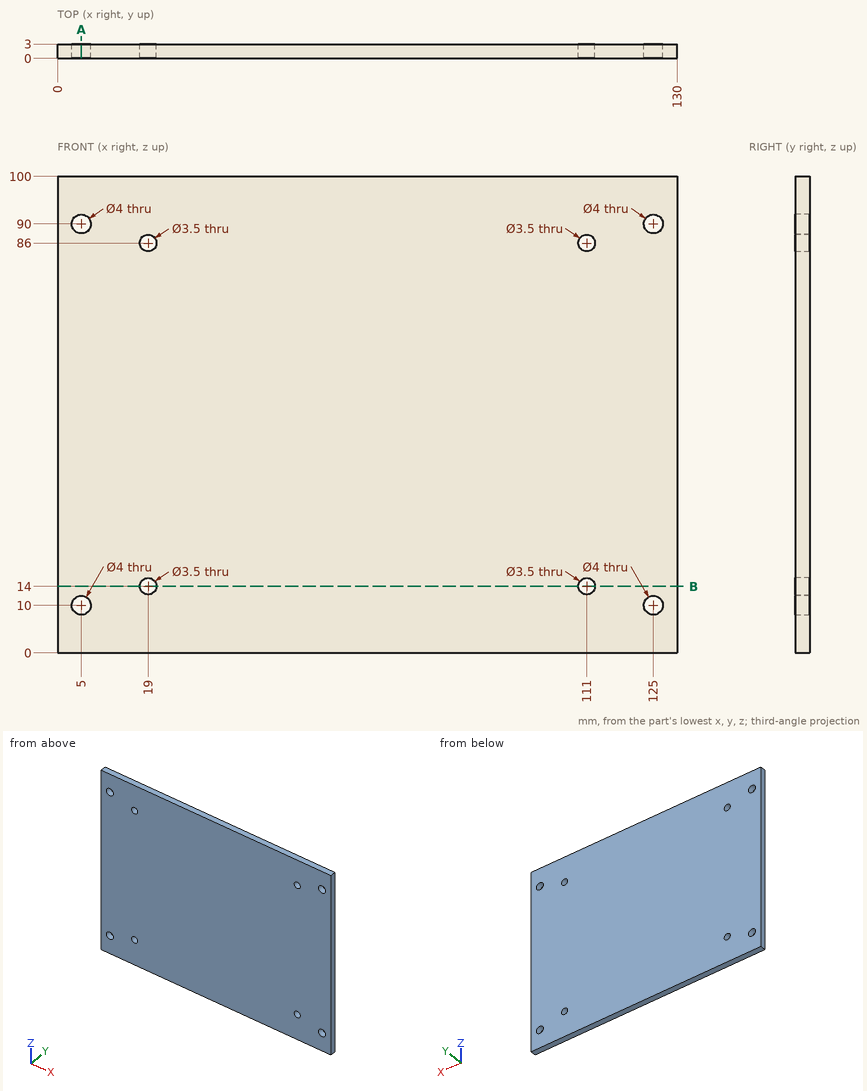
Check sheet for the drawn part. Datum: minimum x, y, z corner. Units: mm. Coordinates: 2 decimals unless noted, no trailing zeros. Loops run counter-clockwise (first coordinate to the right, second up) from the corner with the lowest first, then second, coordinate; pieces in that order, holes last. Notation, with made-up numbers: (18, 65.5) -> (59, 65.5) arc R12 cw to (59, 75.5) -> close; hole circle Ø3 at (42.25, 45.25). An arc over 180 degrees is marked (long way). Answer as CSV lines item,"result".
1) Depth check by flat-ended pin: pin 1 (2.5 mm diameter, centred on x = 5, z = 10, fed in from -Y); pin 2 (4.5 mm diameter, centred on x = 111, z = 14, fed in from +Y). Enter the tip coordinate at first touch or a pass-through.
Found:
pin 1,"passes through"
pin 2,"stops at y = 3"
2) Cross-section at A-A, the plane x = 5. Record the cut outline in (y, z), then the cut area to 3 significant figures.
Found:
outline,"(0, 0) -> (3, 0) -> (3, 8) -> (0, 8) -> close; (0, 12) -> (3, 12) -> (3, 88) -> (0, 88) -> close; (0, 92) -> (3, 92) -> (3, 100) -> (0, 100) -> close"
area,"276 mm2"
3) Thickness scan on L1, parallel to X at y = 0.8, z = 90; L2, parallel to X at y = 1.35, z = 86; L3, parallel to Z at x = 125, y = 1.4. Record the ranges inside material, lowest first. Write a range as from..to.
Found:
L1,"x = 0..3, 7..123, 127..130"
L2,"x = 0..17.25, 20.75..109.25, 112.75..130"
L3,"z = 0..8, 12..88, 92..100"
4) Cross-section at B-B, the plane z = 14. Record the cut outline in (x, y), then the cut area to 3 significant figures.
Found:
outline,"(0, 0) -> (17.25, 0) -> (17.25, 3) -> (0, 3) -> close; (20.75, 0) -> (109.25, 0) -> (109.25, 3) -> (20.75, 3) -> close; (112.75, 0) -> (130, 0) -> (130, 3) -> (112.75, 3) -> close"
area,"369 mm2"
